For this review, use the dimensioned drawing (mm, ordinates from the lowest corner) and the shaded views. A direction names the side the tool comes from. Round coordinates to 2 decimals unless told otherwise and drop trailing zeros. Write each loop counter-clockwise with the first axis right and the second up, starting at its lowest first coordinate (ties: lowest second). Pieces come first, ordered by that corner, then holes.
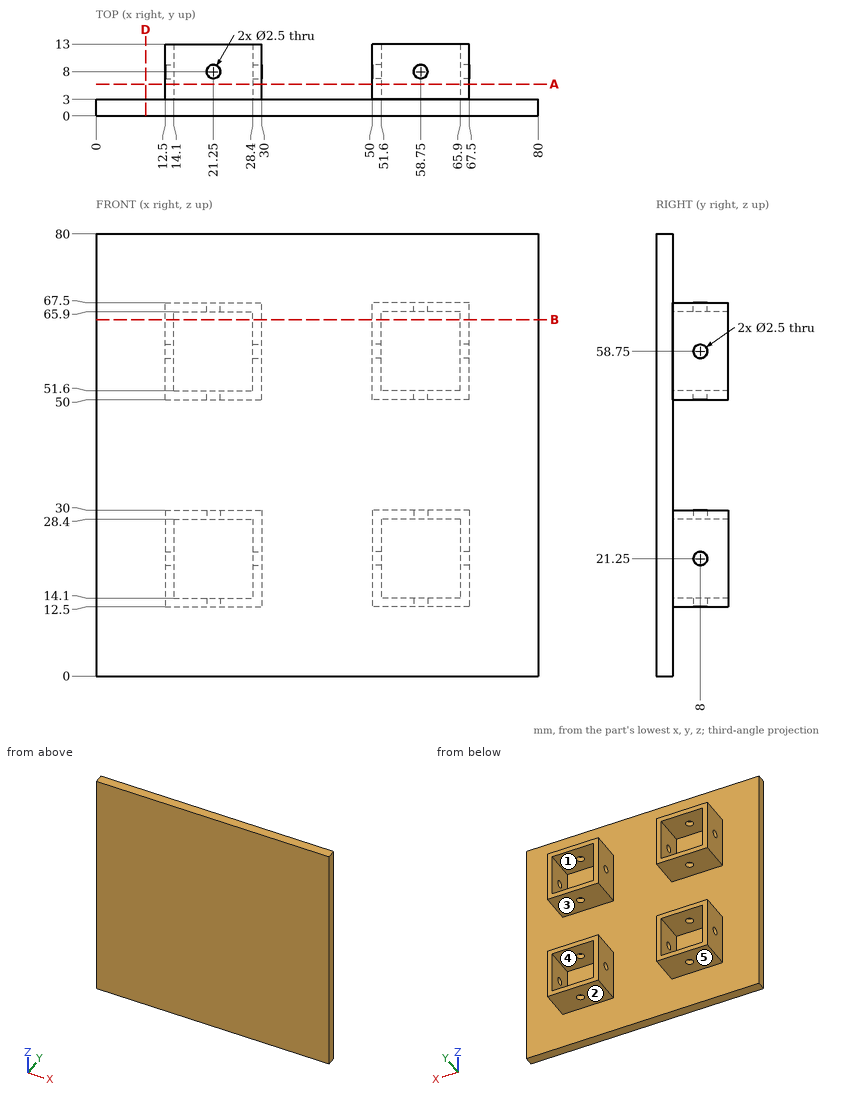
(1) For the marked faces 3, 4 and 5, list the 3-axis set-ups (+Z, -Z, +X, -X, +Y, -Y) from which the entire face can be reached by the end or side of a thin tool; tool diameter is ignored.
Geometry check:
face 3: +X, -X, +Y
face 4: +Y
face 5: -Z, +X, -X, +Y
(2) We need section D-D, the plane x = 9. Give the boundary of the cut face in (y, z), and give its area (3 significant figures).
Geometry check:
outline: (0, 0) - (3, 0) - (3, 80) - (0, 80) - close
area: 240 mm2
(3) We need section B-B, the plane z = 64.5. Give the boundary of the cut face in (x, y), and give its area (3 significant figures).
Geometry check:
outline: (0, 0) - (80, 0) - (80, 3) - (67.5, 3) - (67.5, 13) - (65.9, 13) - (65.9, 3) - (51.6, 3) - (51.6, 13) - (50, 13) - (50, 3) - (30, 3) - (30, 13) - (28.4, 13) - (28.4, 3) - (14.1, 3) - (14.1, 13) - (12.5, 13) - (12.5, 3) - (0, 3) - close
area: 304 mm2
(4) For line 1 along Z through (x, y) = (24.5, 8.5); line 2 along Y through (x, z) = (58.75, 50.6), list the stretches that pass through material, from the lowest coordinate up.
Geometry check:
line 1: z = 12.5 to 14.1, 28.4 to 30, 50 to 51.6, 65.9 to 67.5
line 2: y = 0 to 6.75, 9.25 to 13
(5) Mouldability with a two-part tool opening along X and no side actions: class the marked faces 1 and 2 as pulls with the +X half, pulls with the -X half, needs draft (parallel to the pull), parting line crosses it, or undercut.
Geometry check:
face 1: undercut
face 2: needs draft
(6) For pin 1 Ø5 at (x, y) = (22.5, 10) entering from -Z; pin 2 Ø6 at (y, z) = (6.5, 55.5) entering from +X; pin 3 Ø3 at (x, y) = (56.5, 7.5) entering from +Z, all flat-tipped, find the tip position at first contact; note any pin that passes through.
Geometry check:
pin 1: stops at z = 12.5
pin 2: stops at x = 67.5
pin 3: stops at z = 67.5
(7) We need section A-A, the plane y = 5.75. State how many separate pieces and enclosed holes the cut face has, and give its area (3 significant figures).
Geometry check:
separate pieces: 4
enclosed holes: 4
area: 407 mm2
